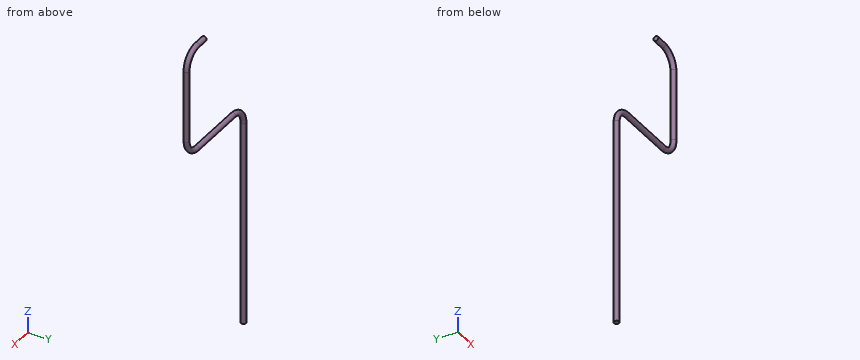
```python
from build123d import *

# Parameters (mm, degrees)
BARRER2_PROFILE_R = 1.5


with BuildPart() as part:
    # Barrer2: sweep along a path in Croquis1
    with BuildLine(Plane(origin=(0, 0, 0), x_dir=(1, 0, 0), z_dir=(0, 1, 0))) as barrer2_path:
        Line((0, 0), (0, -121.77))
        ThreePointArc((0, -121.77), (2.928932188, -128.841067812), (10, -131.77))
        Line((10, -131.77), (45, -131.77))
        ThreePointArc((45, -131.77), (52.071067812, -134.698932188), (55, -141.77))
        Line((55, -141.77), (55, -184.29))
        ThreePointArc((55, -184.29), (52.071067812, -191.361067812), (45, -194.29))
        Line((45, -194.29), (38, -194.29))
    # Barrer2 profile (on start of the path) → Barrer2 (sweep)
    with BuildSketch(Plane.XY):
        Circle(BARRER2_PROFILE_R)
    sweep(path=barrer2_path.line)


solid = part.part
```
For this review, take the finished solid that the model builds, in its own axes (mm). Give positions to 0.01 mm unless a question says otherwise; leave off trailing zeros. Order: outer loops, then holes, each group sorted by start corner. A loop starts at its lowest first (then second) coordinate and runs counter-clockwise, first axis right, second up.
1) Take a section at A-A (x = 41). Give the boundary of the cut face in (y, z), then the cut area to 3 significant figures.
2) Insertion check: pin 1 (1 mm diameter, centred on x = 26, y = 0.5, fed in from -Z). The pin has a flat end and moves straight along its axis. Give the tip position at first contact, or say it passes through.
3) Take a section at B-B (y = 0). Give the boundary of the cut face in (x, z), then the cut area to 3 significant figures.
4) Wall thickness on line 1 (X direction, y = -0.25, z = 90); line 2 (Z direction, x = 16, y = 0.05); line 3 (Z direction, x = 49, y = 1.1): over which ranges is each line inside the solid? List them lowest first.
5) Take a section at C-C (x = 21). Give the boundary of the cut face in (y, z).
Derived:
1. outline: circle Ø3 at (0, 131.77); circle Ø3 at (0, 194.29)
1. area: 14.1 mm2
2. pin 1: stops at z = 130.27
3. outline: (-1.5, 0) - (1.5, 0) - (1.5, 121.77) arc R8.5 cw to (10, 130.27) - (45, 130.27) arc R11.5 ccw to (56.5, 141.77) - (56.5, 184.29) arc R11.5 ccw to (45, 195.79) - (38, 195.79) - (38, 192.79) - (45, 192.79) arc R8.5 cw to (53.5, 184.29) - (53.5, 141.77) arc R8.5 cw to (45, 133.27) - (10, 133.27) arc R11.5 ccw to (-1.5, 121.77) - close
3. area: 760 mm2
4. line 1: x = -1.48 to 1.48
4. line 2: z = 130.27 to 133.27
4. line 3: z = 131.5 to 133.73, 192.33 to 194.56
5. outline: circle Ø3 at (0, 131.77)
